For this review, use the dimensioned drawing (mm, ordinates from the lowest corner) and the shaded views. A direction names the side the tool comes from. Round coordinates to 2 decimals unless told otherwise and drop trailing zeros. Loops run counter-clockwise (first coordinate to the right, second up) from the corner with the lowest first, then second, coordinate; pieces in that order, holes last. Notation, with made-up numbers: (-9.5, 38.5) -> (12.5, 38.5) arc R11 cw to (12.5, 54.5) -> close; hole circle Ø10 at (75.5, 89.5). An arc over 180 degrees is marked (long way). Use one line per item in the form item = value. Start each with the question number.
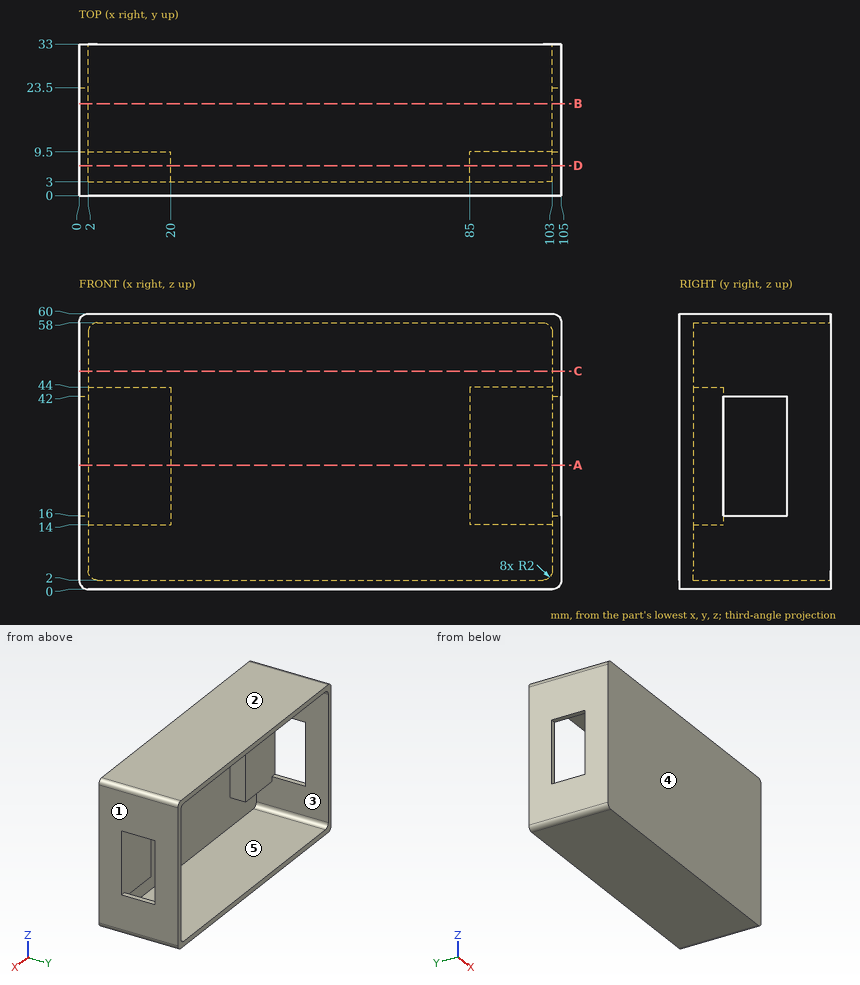
Item 1: For P1, Ø8, axis at x = 14, z = 11, coming from the +Y side, flat-tipped, find the tip position at first contact; note if it passes through.
Item 2: Take a section at D-D on y = 6.5. Give the boundary of the cut face in (x, z).
Item 3: Draft analysis for pull direction X (two halves, no side actions). For the marked faces 1, 2 and 3, state which applies: +X half, -X half, draft (parallel to the pull), parting line (faces both ways), or undercut.
Item 4: Wall thickness on line 1 (Z direction, x = 18, y = 23.5); line 2 (X direction, y = 7, z = 42.5); line 3 (X direction, y = 7, z = 48): over which ranges is each line inside the solid? List them lowest first.
Item 5: Take a section at C-C on z = 47.5. Give the boundary of the cut face in (x, y), plus the area to 3 significant figures.
Item 6: Take a section at A-A on z = 27. Give the boundary of the cut face in (x, y).
Item 7: Machinability: for the marked faces 4 and 5, which of the approach directions +Z, -Z, +X, -X, +Y, -Y give a long, thin tool a straight path to every point of the face, cutting with its end or side? Answer none if there is none.
Item 8: Take a section at B-B on y = 20. Give the boundary of the cut face in (x, z), plus the area to 3 significant figures.
Results:
q1.P1 = 9.5
q2.outline = (0, 2) arc R2 ccw to (2, 0) -> (103, 0) arc R2 ccw to (105, 2) -> (105, 58) arc R2 ccw to (103, 60) -> (2, 60) arc R2 ccw to (0, 58) -> close; hole (2, 4) arc R2 ccw to (4, 2) -> (101, 2) arc R2 ccw to (103, 4) -> (103, 14) -> (85, 14) -> (85, 44) -> (103, 44) -> (103, 56) arc R2 ccw to (101, 58) -> (4, 58) arc R2 ccw to (2, 56) -> (2, 44) -> (20, 44) -> (20, 14) -> (2, 14) -> close
q3.face_1 = +X half
q3.face_2 = draft
q3.face_3 = undercut
q4.line_1 = 0 to 2, 58 to 60
q4.line_2 = 0 to 20, 85 to 105
q4.line_3 = 0 to 2, 103 to 105
q5.outline = (0, 0) -> (105, 0) -> (105, 33) -> (103, 33) -> (103, 3) -> (2, 3) -> (2, 33) -> (0, 33) -> close
q5.area = 435 mm2
q6.outline = (0, 0) -> (105, 0) -> (105, 9.5) -> (85, 9.5) -> (85, 3) -> (20, 3) -> (20, 9.5) -> (0, 9.5) -> close; (0, 23.5) -> (2, 23.5) -> (2, 33) -> (0, 33) -> close; (103, 23.5) -> (105, 23.5) -> (105, 33) -> (103, 33) -> close
q7.face_4 = +Z, -Z, +X, -X, -Y
q7.face_5 = +Y
q8.outline = (0, 2) arc R2 ccw to (2, 0) -> (103, 0) arc R2 ccw to (105, 2) -> (105, 16) -> (103, 16) -> (103, 4) arc R2 cw to (101, 2) -> (4, 2) arc R2 cw to (2, 4) -> (2, 16) -> (0, 16) -> close; (0, 42) -> (2, 42) -> (2, 56) arc R2 cw to (4, 58) -> (101, 58) arc R2 cw to (103, 56) -> (103, 42) -> (105, 42) -> (105, 58) arc R2 ccw to (103, 60) -> (2, 60) arc R2 ccw to (0, 58) -> close
q8.area = 540 mm2
